The listing builds one solid part. Answer for the finished solid, in the listing's coordinates (mm). A direction names the side the tool comes from. Give positions to 0.01 mm unless a question says otherwise; leave off trailing zeros. Order: outer loops, then holes, each group sorted by start corner. A loop starts at its lowest first (then second) coordinate and runs counter-clockwise, first axis right, second up. Notation, with made-up numbers: (46.5, 56.5) - (82.5, 56.5) arc R28 ccw to (82.5, 80.5) - close; hole circle Ø8 at (-21.75, 33.5). An arc over 180 degrees is marked (long way). Answer as a JSON object with one key per item and string values. Group by question number.
Q1. Consider line 1 (Z direction, x = 0, y = 1.55); line 2 (Z direction, x = -2, y = -0.75); line 3 (Z direction, x = -3.5, y = 1.5). Determine where each line is inside the solid, lowest interval first.
Q2. Given pin 1 (0.9 mm diameter, centred on y = -0.5, z = 5.5, fed in from -X); pin 2 (1.5 mm diameter, centred on y = -2, z = -10, fed in from -X); pin 3 (5 mm diameter, centred on x = 0, z = 8.5, fed in from +Y), each flat-ended and moving along its own axis, determine where each tip first touches the part or whether it passes through.
Q3. A cutting plane is placed at C-C, the plane z = -6.25. Give the vertices of the cut face in (x, y).
Q4. A cutting plane is placed at D-D, the plane x = 4.75. Give the vertices of the cut face in (y, z).
Q5. A cutting plane is placed at B-B, the plane z = 7.5. Give the vertices of the cut face in (x, y).
Q6. For faces 5 (the face through (1.9, 0.08, -6.34)), 6 (the face through (-2.199, -2.215, 6.219)), 7 (the face through (0, 2.5, 6)), 8 (the face through (2.199, -2.215, 6.282)), 9 (the face through (0, -4, 3)), determine the directions among +Z, -Z, +X, -X, +Y, -Y from which every point of the face is accessible in a straight line to the end or side of a thin tool.
Q7. The mould has two halves that part along X. Classify faces 1 (the face through (-1.08, 4.88, 1.48)), 2 (the face through (-2.215, 2.199, 6.219)), 3 (the face through (2.215, 2.199, 6.282)), 4 (the face through (-2, 1, -12.5)): released by +X, released by -X, zero draft, split by the parting line, or undercut.
Autodesk Inventor part; units mm, degrees
ref_plane "작업 평면1" through (0, 0, 0) normal (0, 1, 0) x (-1, 0, 0)
ref_plane "작업 평면2" through (0, 0, -12.5) normal (0, 0, -1) x (-1, 0, 0)
ref_plane "YZ Plane" through (0, 0, 0) normal (1, 0, 0) x (0, 1, 0)
sketch "스케치1" plane through (0, 0, 0) normal (0, 0, 1) x (1, 0, 0)
  circle A0 centre (0, 0) radius 5
  dimension "d0" = 10
extrude "돌출1" add sketch "스케치1" along normal blind 3
ref_plane "작업 평면1" through (0, 0, 0) normal (0, 1, 0) x (-1, 0, 0)
sketch "스케치2" plane through (0, 0, 0) normal (0, 1, 0) x (-1, 0, 0)
  line L0 (5, 3) -> (-5, 3)
  line L1 (2.5, 3) -> (-2.5, 3)
  line L2 (-2.5, 3) -> (-2.5, 11)
  line L3 (-2.5, 11) -> (2.5, 11)
  line L4 (2.5, 11) -> (2.5, 3)
  circle A0 centre (0, 8.5) radius 1.5
  point P0 (0, 0)
  point P1 (0, 3)
  point P2 (0, 11)
  dimension "d3" = 5
  dimension "d4" = 8
  dimension "d5" = 3
  dimension "d15" = 2.5
extrude "돌출2" add sketch "스케치2" along normal mid plane 5
fillet "모깎기1" radius 2.5 2 edges at (2.5, 0, 11) (-2.5, 0, 11)
fillet "모깎기2" radius 1 6 edges at (1.7679, 2.5, 10.2679) (2.5, 2.5, 5.7503) (-2.5, 2.5, 5.7503) (1.7679, -2.5, 10.2679) (2.5, -2.5, 5.7503) (-2.5, -2.5, 5.7503)
fillet "모깎기3" radius 1 8 edges at (-2.2073, -2.2073, 3) (-2.5, 0, 3) (-2.2073, 2.2073, 3) (0, 2.5, 3) (2.2073, 2.2073, 3) (2.5, 0, 3) (2.2073, -2.2073, 3) (0, -2.5, 3)
sketch "스케치3" plane through (0, 0, 0) normal (0, 0, -1) x (-1, 0, 0)
  circle A0 centre (0, 0) radius 4
  circle A1 centre (0, 0) radius 2.5
  dimension "d11" = 8
  dimension "d12" = 5
extrude "돌출3" add sketch "스케치3" along normal blind 15 contours A1
ref_plane "작업 평면2" through (0, 0, -12.5) normal (0, 0, -1) x (-1, 0, 0)
sketch "스케치4" plane through (0, 0, -12.5) normal (0, 0, -1) x (-1, 0, 0)
  circle A0 centre (0, 0) radius 1.9
  circle A1 centre (0, 0) radius 2.5
  circle A2 centre (0, 0) radius 2.5
  dimension "d17" = 3.8
extrude "돌출4" cut sketch "스케치4" against normal up to surface (12.5 mm away)
properties part number "SuspensionBase"
Reply:
{
 "1": {"line 1": "z = -15 to 7, 10 to 11", "line 2": "z = -15 to -12.5, 0 to 10", "line 3": "z = 0 to 3"},
 "2": {"pin 1": "stops at x = -2.5", "pin 2": "stops at x = -1.43", "pin 3": "stops at y = 2.5"},
 "3": {"outline": "circle Ø3.8 at (0, 0)"},
 "4": {"outline": "(-1.56, 0) - (1.56, 0) - (1.56, 3) - (-1.56, 3) - close"},
 "5": {"outline": "(-2.5, -1.5) arc R1 ccw to (-1.5, -2.5) - (-1.12, -2.5) - (-1.12, 2.5) - (-1.5, 2.5) arc R1 ccw to (-2.5, 1.5) - close; (1.12, -2.5) - (1.5, -2.5) arc R1 ccw to (2.5, -1.5) - (2.5, 1.5) arc R1 ccw to (1.5, 2.5) - (1.12, 2.5) - close"},
 "6": {"face 5": "none", "face 6": "+Z, -X, -Y", "face 7": "+Z, +X, -X, +Y", "face 8": "+Z, +X, -Y", "face 9": "+Z"},
 "7": {"face 1": "split by the parting line", "face 2": "released by -X", "face 3": "released by +X", "face 4": "zero draft"}
}
